from build123d import *

# Parameters (mm, degrees)
SKETCH1_W           = 50.8
SKETCH1_H           = 50.8
SKETCH1_R           = 12.7
BOSS_EXTRUDE1_DEPTH = 12.7
SKETCH2_R           = 28.398063314
SKETCH2_R_2         = 22.86
BOSS_EXTRUDE2_DEPTH = 254
SCALE1_SCALE        = 3
SCALE2_SCALE        = 0.333333333
SCALE3_SCALE        = 2


with BuildPart() as part:
    # Sketch1 → Boss-Extrude1 (new body)
    with BuildSketch(Plane(origin=(0, 0, 0), x_dir=(1, 0, 0), z_dir=(0, 1, 0))):
        with Locations((25.4, 25.4)):
            Rectangle(SKETCH1_W, SKETCH1_H)
        with Locations(Location((25.4, 25.4, 0), (0, 0, 270))):
            Circle(SKETCH1_R, mode=Mode.SUBTRACT)
    extrude(amount=BOSS_EXTRUDE1_DEPTH)

    # Sketch2 → Boss-Extrude2 (add)
    with BuildSketch(Plane(origin=(50.8, 0, 0), x_dir=(0, 0, -1), z_dir=(1, 0, 0))):
        with Locations(Location((25.4, 12.7, 0), (0, 0, 206.565051177))):
            Circle(SKETCH2_R)
        with Locations((25.4, 12.7)):
            Circle(SKETCH2_R_2, mode=Mode.SUBTRACT)
    extrude(amount=BOSS_EXTRUDE2_DEPTH)


with BuildPart() as part_1:
    # Scale1: scaled about (161.925226112, 12.038551088, -25.4)
    add(part.part.scale(SCALE1_SCALE).moved(Location((-323.850452224, -24.077102176, 50.8))))


with BuildPart() as part_2:
    # Scale2: scaled about (161.925226113, 12.038551088, -25.4)
    add(part_1.part.scale(SCALE2_SCALE).moved(Location((107.950150742, 8.025700725, -16.933333333))))


with BuildPart() as part_3:
    # Scale3: scaled about (161.925226113, 12.038551088, -25.4)
    add(part_2.part.scale(SCALE3_SCALE).moved(Location((-161.925226113, -12.038551088, 25.4))))


solid = part_3.part
Source: CAD feature listing. Evaluate the final solid. Frame: model axes, mm. A direction names the side the tool comes from. Give positions to 0.01 mm unless a question says otherwise; leave off trailing zeros. Write each loop counter-clockwise with the first axis right and the second up, starting at its lowest first coordinate (ties: lowest second). Pieces come first, ordered by that corner, then holes. Notation, with made-up numbers: M 35,1.25 L 75,1.25 A22 ccw 75,36.25 Z; hole C 62.25,58.25 d7. An arc over 180 degrees is marked long. Return JSON: item names as keys, results as strings. Group by question number.
1) Set-up query: faces 1 (the face through (-112, 0, -76.2)), 2 (the face through (-134, -12.039, -37)), 3 (the face through (-112, 0, 25.4)), 4 (the face through (-134, 13.361, -37)). Return all of +Z, -Z, +X, -X, +Y, -Y with unobstructed straight access to the full face (end or side cutting, diameter ignored); none if empty.
2) Cut plane A-A, the plane z = -25.4. Output: boundary loops of the cut face in (x, y), then the cut area to 3 significant figures.
3) First-contact query: pin 1 Ø12.5 at (x, y) = (-124, 2.5) entering from +Z; pin 2 Ø12 at (y, z) = (13.5, -11) entering from -X; pin 3 Ø5 at (x, z) = (159, -9.5) entering from -Y; pin 4 Ø1 at (x, z) = (338, -37.5) entering from -Y. Flat tips, straight axial feed; report the tip coordinate or a pass-through.
4) Ray query, L1, parallel to X at y = -4.75, z = -25.4; L2, parallel to Y at x = 168, z = -25; L3, parallel to Z at x = 157.5, y = 13. Return the intervals inside material, ascending.
5) Cut plane B-B, the plane y = 4.5. Output: boundary loops of the cut face in (x, z).
6) Cut plane C-C, the plane x = 184. Output: boundary loops of the cut face in (y, z).
7) Draft query along Y for faces 5 (the face through (190.12, -2.25, -80.01)), 6 (the face through (-60.325, 0, -25)), 7 (the face through (447.675, 8, -71)). Return one class per face: released by +Y, released by -Y, zero draft, split by the parting line, or undercut.
Data:
{
 "1": {"face 1": "-Z, -X, +Y, -Y", "face 2": "+Z, -Z, -X, -Y", "face 3": "+Z, -X, +Y, -Y", "face 4": "+Z, -Z, -X, +Y"},
 "2": {"outline": "M -161.93,-12.04 L -136.53,-12.04 L -136.53,13.36 L -161.93,13.36 Z; M -85.73,-12.04 L -60.33,-12.04 L -60.33,13.36 L -85.73,13.36 Z; M -60.33,-43.43 L 447.67,-43.43 L 447.67,-32.36 L -60.33,-32.36 Z; M -60.33,59.08 L 447.67,59.08 L 447.67,70.16 L -60.33,70.16 Z", "area": "12,500 mm²"},
 "3": {"pin 1": "stops at z = 25.4", "pin 2": "stops at x = -161.93", "pin 3": "stops at y = -41.83", "pin 4": "stops at y = -42.24"},
 "4": {"L1": "x = -161.93 to -136.53, -85.73 to -60.33", "L2": "y = -43.43 to -32.36, 59.08 to 70.16", "L3": "z = -82.19 to -71.12, 20.32 to 31.39"},
 "5": {"outline": "M -161.93,-76.2 L -60.33,-76.2 L -60.33,-81.5 L 447.67,-81.5 L 447.67,-70.25 L -60.33,-70.25 L -60.33,19.45 L 447.67,19.45 L 447.67,30.7 L -60.33,30.7 L -60.33,25.4 L -161.93,25.4 Z; hole C -111.13,-25.4 d50.8"},
 "6": {"outline": "C 13.36,-25.4 d113.59; hole C 13.36,-25.4 d91.44"},
 "7": {"face 5": "split by the parting line", "face 6": "undercut", "face 7": "zero draft"}
}
